Design review of the part built by this model. Coordinates are the model's own, in mm. A direction names the side the tool comes from. Coordinates: 2 decimals unless noted, no trailing zeros. Loops run counter-clockwise (first coordinate to the right, second up) from the corner with the lowest first, then second, coordinate; pieces in that order, holes last.
from build123d import *
from OCP.BRepFilletAPI import BRepFilletAPI_MakeChamfer

# Parameters (mm, degrees)
SKETCH1_W                 = 40.5
SKETCH1_H                 = 20
BOSS_EXTRUDE1_DEPTH       = 37.75
SKETCH2_W                 = 2.75
SKETCH2_H                 = 18
BOSS_EXTRUDE2_DEPTH       = 8
SKETCH3_R                 = 2
CUT_EXTRUDE1_DEPTH        = 4
SKETCH4_W                 = 3.75
SKETCH4_H                 = 1.5
BOSS_EXTRUDE3_DEPTH       = 1.25
CHAMFER1_SIZE2            = 0.865755717
CHAMFER1_SIZE             = 3.75
CHAMFER2_SIZE             = 0.25
CHAMFER2_SIZE2            = 0.333581356
FILLET1_R                 = 0.25
CHAMFER1_OF_MIRROR1_SIZE2 = 0.865755717
CHAMFER1_OF_MIRROR1_SIZE  = 3.75
CHAMFER2_OF_MIRROR1_SIZE2 = 0.25
CHAMFER2_OF_MIRROR1_SIZE  = 0.333581356
FILLET1_OF_MIRROR1_R      = 0.25
SKETCH5_W                 = 11.3
SKETCH5_H                 = 17
BOSS_EXTRUDE4_DEPTH       = 1
SKETCH6_R                 = 6
BOSS_EXTRUDE5_DEPTH       = 1.5
CHAMFER3_SIZE2            = 0.866025404
CHAMFER3_SIZE             = 1.5
SKETCH7_R                 = 3
SKETCH7_R_2               = 0.75
BOSS_EXTRUDE6_DEPTH       = 4.25
SKETCH8_W                 = 3.25
SKETCH8_H                 = 7.25
SKETCH8_W_2               = 1.25
SKETCH8_H_2               = 5.25
BOSS_EXTRUDE7_DEPTH       = 2.5
CHAMFER5_SIZE2            = 3.575260778
CHAMFER5_SIZE             = 3
CHAMFER4_SIZE             = 2.5
CHAMFER4_SIZE_2           = 0.669872981
FILLET2_R                 = 0.5


with BuildPart() as part:
    # Sketch1 → Boss-Extrude1 (new body)
    with BuildSketch(Plane.XY):
        Rectangle(SKETCH1_W, SKETCH1_H)
    extrude(amount=BOSS_EXTRUDE1_DEPTH)

    # Sketch2 → Boss-Extrude2 (add)
    with BuildSketch(Plane(origin=(20.25, 0, 0), x_dir=(0, 0, -1), z_dir=(1, 0, 0))):
        with Locations((-29.375, 0)):
            Rectangle(SKETCH2_W, SKETCH2_H)
    boss_extrude2 = extrude(amount=BOSS_EXTRUDE2_DEPTH)

    # Sketch3 → Cut-Extrude1 (cut)
    with BuildSketch(Plane.XY.offset(30.75)):
        with Locations((24.25, 5)):
            Circle(SKETCH3_R)
        with Locations((24.25, -5)):
            Circle(SKETCH3_R)
    cut_extrude1 = extrude(amount=-CUT_EXTRUDE1_DEPTH, mode=Mode.SUBTRACT)

    # Sketch4 → Boss-Extrude3 (add)
    with BuildSketch(Plane.XY.offset(30.75)):
        with Locations((22.125, 0)):
            Rectangle(SKETCH4_W, SKETCH4_H)
    boss_extrude3 = extrude(amount=BOSS_EXTRUDE3_DEPTH)

    # Chamfer1
    chamfer1_edges = [part.edges().sort_by_distance(p)[0] for p in [
        (24, 0, 32),
    ]]
    chamfer1_side = [part.faces().sort_by_distance(p)[0] for p in [
        (23.982684886, 0, 32),
    ]]
    chamfer(chamfer1_edges, length=CHAMFER1_SIZE - 0.0001, length2=CHAMFER1_SIZE2 - 0.0001, reference=chamfer1_side[0])  # a hair under: the kernel refuses the full size

    # Chamfer2
    chamfer2_edges = [part.edges().sort_by_distance(p)[0] for p in [
        (24, 0, 31.134344283),
    ]]
    chamfer2_side = [part.faces().sort_by_distance(p)[0] for p in [
        (22.12505, 0, 31.567172141),
    ]]
    chamfer(chamfer2_edges, length=CHAMFER2_SIZE, length2=CHAMFER2_SIZE2, reference=chamfer2_side[0])

    # Fillet1
    fillet1_edges = [part.edges().sort_by_distance(p)[0] for p in [
        (24.25, 9, 30.75),
        (24.25, -9, 30.75),
        (24.25, -9, 28),
        (24.25, 9, 28),
        (28.25, 0, 30.75),
        (28.25, -9, 29.375),
        (28.25, 0, 28),
        (28.25, 9, 29.375),
    ]]
    fillet(fillet1_edges, radius=FILLET1_R)

    # Mirror1: Boss-Extrude2, Cut-Extrude1, Boss-Extrude3 across plane
    add(boss_extrude2.mirror(Plane(origin=(0, 0, 0), x_dir=(0, 0, 1), z_dir=(1, 0, 0))))
    add(cut_extrude1.mirror(Plane(origin=(0, 0, 0), x_dir=(0, 0, 1), z_dir=(1, 0, 0))), mode=Mode.SUBTRACT)
    add(boss_extrude3.mirror(Plane(origin=(0, 0, 0), x_dir=(0, 0, 1), z_dir=(1, 0, 0))))

    # Chamfer1 of Mirror1
    chamfer1_of_mirror1_edges = [part.edges().sort_by_distance(p)[0] for p in [
        (-24, 0, 32),
    ]]
    chamfer1_of_mirror1_side = [part.faces().sort_by_distance(p)[0] for p in [
        (-23.982684886, 0, 32),
    ]]
    chamfer(chamfer1_of_mirror1_edges, length=CHAMFER1_OF_MIRROR1_SIZE - 0.0001, length2=CHAMFER1_OF_MIRROR1_SIZE2 - 0.0001, reference=chamfer1_of_mirror1_side[0])  # a hair under: the kernel refuses the full size

    # Chamfer2 of Mirror1
    chamfer2_of_mirror1_edges = [part.edges().sort_by_distance(p)[0] for p in [
        (-24, 0, 31.134344283),
    ]]
    chamfer(chamfer2_of_mirror1_edges, length=CHAMFER2_OF_MIRROR1_SIZE, length2=CHAMFER2_OF_MIRROR1_SIZE2)

    # Fillet1 of Mirror1
    fillet1_of_mirror1_edges = [part.edges().sort_by_distance(p)[0] for p in [
        (-24.25, 9, 30.75),
        (-24.25, -9, 30.75),
        (-24.25, -9, 28),
        (-24.25, 9, 28),
        (-28.25, 0, 30.75),
        (-28.25, -9, 29.375),
        (-28.25, 0, 28),
        (-28.25, 9, 29.375),
    ]]
    fillet(fillet1_of_mirror1_edges, radius=FILLET1_OF_MIRROR1_R)

    # Sketch5 → Boss-Extrude4 (add)
    with BuildSketch(Plane.XY.offset(37.75)):
        with Locations((11.6, 0)):
            Rectangle(SKETCH5_W, SKETCH5_H)
    extrude(amount=BOSS_EXTRUDE4_DEPTH)

    # Sketch6 → Boss-Extrude5 (add)
    with BuildSketch(Plane.XY.offset(37.75)):
        with Locations(Location((-10.25, 0, 0), (0, 0, 180))):
            Circle(SKETCH6_R)
    extrude(amount=BOSS_EXTRUDE5_DEPTH)

    # Chamfer3
    chamfer3_edges = [part.edges().sort_by_distance(p)[0] for p in [
        (-4.25, 0, 39.25),
    ]]
    chamfer3_side = [part.faces().sort_by_distance(p)[0] for p in [
        (-4.25, 0, 39.232679492),
    ]]
    chamfer(chamfer3_edges, length=CHAMFER3_SIZE - 0.0001, length2=CHAMFER3_SIZE2 - 0.0001, reference=chamfer3_side[0])  # a hair under: the kernel refuses the full size

    # Sketch7 → Boss-Extrude6 (add)
    with BuildSketch(Plane.XY.offset(39.25)):
        with Locations((-10.25, 0)):
            Circle(SKETCH7_R)
        with Locations((-10.25, 0)):
            Circle(SKETCH7_R_2, mode=Mode.SUBTRACT)
    extrude(amount=BOSS_EXTRUDE6_DEPTH)

    # Sketch8 → Boss-Extrude7 (add)
    with BuildSketch(Plane.ZY.offset(20.25)):
        with Locations((3.125, 0)):
            Rectangle(SKETCH8_W, SKETCH8_H)
        with Locations((3.125, 0)):
            Rectangle(SKETCH8_W_2, SKETCH8_H_2, mode=Mode.SUBTRACT)
    extrude(amount=BOSS_EXTRUDE7_DEPTH)

    # Chamfer5
    chamfer5_edges = [part.edges().sort_by_distance(p)[0] for p in [
        (20.25, 0, 37.75),
    ]]
    chamfer5_side = [part.faces().sort_by_distance(p)[0] for p in [
        (20.19, 0, 37.75),
    ]]
    chamfer(chamfer5_edges, length=CHAMFER5_SIZE - 0.0001, length2=CHAMFER5_SIZE2 - 0.0001, reference=chamfer5_side[0])  # a hair under: the kernel refuses the full size

    # Chamfer4
    chamfer4_edges_1 = [part.edges().sort_by_distance(p)[0] for p in [
        (-22.75, -3.625, 3.125),
    ]]
    chamfer4_side_1 = [part.faces().sort_by_distance(p)[0] for p in [
        (-22.73660254, -3.625, 3.125),
    ]]
    chamfer4_edges_2 = [part.edges().sort_by_distance(p)[0] for p in [
        (-22.75, 0, 4.75),
    ]]
    chamfer4_side_2 = [part.faces().sort_by_distance(p)[0] for p in [
        (-22.73660254, 0, 4.75),
    ]]
    chamfer4_edges_3 = [part.edges().sort_by_distance(p)[0] for p in [
        (-22.75, 3.625, 3.125),
    ]]
    chamfer4_side_3 = [part.faces().sort_by_distance(p)[0] for p in [
        (-22.73660254, 3.625, 3.125),
    ]]
    chamfer4_edges_4 = [part.edges().sort_by_distance(p)[0] for p in [
        (-22.75, 0, 1.5),
    ]]
    chamfer4_side_4 = [part.faces().sort_by_distance(p)[0] for p in [
        (-22.73660254, 0, 1.5),
    ]]
    chamfer4 = BRepFilletAPI_MakeChamfer(part.part.solid().wrapped)
    for e in chamfer4_edges_1:
        chamfer4.Add(CHAMFER4_SIZE - 0.0001, CHAMFER4_SIZE_2 - 0.0001, e.wrapped, chamfer4_side_1[0].wrapped)
    for e in chamfer4_edges_2:
        chamfer4.Add(CHAMFER4_SIZE - 0.0001, CHAMFER4_SIZE_2 - 0.0001, e.wrapped, chamfer4_side_2[0].wrapped)
    for e in chamfer4_edges_3:
        chamfer4.Add(CHAMFER4_SIZE - 0.0001, CHAMFER4_SIZE_2 - 0.0001, e.wrapped, chamfer4_side_3[0].wrapped)
    for e in chamfer4_edges_4:
        chamfer4.Add(CHAMFER4_SIZE - 0.0001, CHAMFER4_SIZE_2 - 0.0001, e.wrapped, chamfer4_side_4[0].wrapped)
    add(Compound.cast(chamfer4.Shape()), mode=Mode.REPLACE)  # a hair under: the kernel refuses the full size

    # Fillet2
    fillet2_edges = [part.edges().sort_by_distance(p)[0] for p in [
        (-20.25, 0, 37.75),
        (-1.49995, -10, 37.75),
        (-1.49995, 10, 37.75),
        (20.25, 10, 17.087419611),
        (18.75005, 10, 35.962419611),
        (20.25, -10, 17.087419611),
        (18.75005, -10, 35.962419611),
        (0, -10, 0),
        (-20.25, 0, 0),
        (0, 10, 0),
        (20.25, 0, 0),
        (-20.25, -10, 18.875),
        (-20.25, 10, 18.875),
    ]]
    fillet(fillet2_edges, radius=FILLET2_R)


solid = part.part
Q1. Machinability: for faces 5 (the flat face through (-21, -2.625, 3)), 6 (the flat face through (-14, 0, 39.25)), 7 (the flat face through (-21.52, -0.05, 4.41)), which of the approach directions +Z, -Z, +X, -X, +Y, -Y give a long, thin tool a straight path to every point of the face, cutting with its end or side? Answer none if there is none.
Q2. For line 1 (Y direction, x = 24.25, z = 29.55); line 2 (Y direction, x = -10.25, z = 40.95); line 3 (X direction, y = 5.25, z = 33.5), list the stretches that pass through material, from the lowest coordinate up.
Q3. The part is to be moulded in two halves that separate along Y. For faces 1 (the flat face through (-20.25, 0, 19)), 2 (the flat face through (-24, 9, 29)), 3 (the flat face through (-20.25, 0, 3)), 4 (the flat face through (-21.518, -3.285, 3.102)), say which applies: pulls with the +Y half, pulls with the -Y half, needs draft (parallel to the pull), parting line crosses it, or undercut.
Q4. Take a section at A-A, the plane x = 16. Write out the cut boundary in (y, z).
Q5. Clearance check with flat-ended pins moving along their axes: pin 1 Ø3 at (x, y) = (-4.5, -3.5) entering from +Z; pin 2 Ø8 at (y, z) = (3.5, 26.5) entering from -X; pin 3 Ø1.8 at (x, z) = (23, 29.5) entering from -Y; pin 4 Ø2.5 at (x, z) = (-23.5, 29) entering from +Y. State where each tip first meets the part, or that it passes through.
Q6. Take a section at B-B, the plane z = 6. Write out the cut boundary in (x, y).
Entries:
1. face 5: -X
1. face 6: +Z
1. face 7: -X, +Y, -Y
2. line 1: y = -9 to -7, -3 to 3, 7 to 9
2. line 2: y = -3 to -0.75, 0.75 to 3
2. line 3: x = -20.25 to 20.25
3. face 1: needs draft
3. face 2: pulls with the +Y half
3. face 3: undercut
3. face 4: pulls with the -Y half
4. outline: (-10, 0.5) arc R0.5 ccw to (-9.5, 0) - (9.5, 0) arc R0.5 ccw to (10, 0.5) - (10, 37.25) arc R0.5 ccw to (9.5, 37.75) - (8.5, 37.75) - (8.5, 38.75) - (-8.5, 38.75) - (-8.5, 37.75) - (-9.5, 37.75) arc R0.5 ccw to (-10, 37.25) - close
5. pin 1: stops at z = 39.08
5. pin 2: stops at x = -28.25
5. pin 3: stops at y = -9
5. pin 4: stops at y = 9
6. outline: (-20.25, -9.5) arc R0.5 ccw to (-19.75, -10) - (19.75, -10) arc R0.5 ccw to (20.25, -9.5) - (20.25, 9.5) arc R0.5 ccw to (19.75, 10) - (-19.75, 10) arc R0.5 ccw to (-20.25, 9.5) - close
